Build history of the part. All positions in model axes, mm. A direction names the side the tool comes from. Give positions to 0.01 mm unless a question says otherwise; leave off trailing zeros. Order: outer loops, then holes, each group sorted by start corner. A loop starts at its lowest first (then second) coordinate and runs counter-clockwise, first axis right, second up. Notation, with made-up numbers: (42.5, 3.5) - (82.5, 3.5) arc R26 ccw to (82.5, 38.5) - close; hole circle Ø2 at (33.25, -25.5). An arc over 180 degrees is marked (long way). One line per item, written item: value.
```python
from build123d import *

# Parameters (mm, degrees)
F0_W      = 43.3
F0_H      = 33.3
F1_DEPTH  = 10
F2_W      = 40
F2_H      = 30
F3_DEPTH  = 8.5
F4_W      = 25.5
F4_H      = 15
F5_DEPTH  = 25
F4_R      = 0.85
F6_DEPTH  = 4
F7_W      = 43.3
F7_H      = 33.3
F7_W_2    = 41.7
F7_H_2    = 31.7
F8_DEPTH  = 1
F9_R      = 2
F9_R_2    = 1
F10_DEPTH = 5
F12_SIZE  = 1
F13_R     = 1.3


with BuildPart() as f1:
    # F0 (on Top) → F1 (new body)
    with BuildSketch(Plane.XY):
        Rectangle(F0_W, F0_H)
    extrude(amount=F1_DEPTH)

    # F2 (on face) → F3 (cut)
    with BuildSketch(Plane.XY):
        Rectangle(F2_W, F2_H)
    extrude(amount=F3_DEPTH, mode=Mode.SUBTRACT)

    # F4 (on face) → F5 (cut)
    with BuildSketch(Plane(origin=(0, 0, 8.5), x_dir=(1, 0, 0), z_dir=(0, 0, -1))):
        with Locations((0, -2.1)):
            Rectangle(F4_W, F4_H)
    extrude(amount=-F5_DEPTH, mode=Mode.SUBTRACT)

    # F4 (on face) → F6 (join)
    with BuildSketch(Plane(origin=(0, 0, 8.5), x_dir=(1, 0, 0), z_dir=(0, 0, -1))):
        with Locations((12.2893061021, 12)):
            Circle(F4_R)
        with Locations((-12.2893061021, 12)):
            Circle(F4_R)
        with Locations((-12.2893061021, -12)):
            Circle(F4_R)
        with Locations((12.2893061021, -12)):
            Circle(F4_R)
    extrude(amount=F6_DEPTH)

    # F7 (on face) → F8 (join)
    with BuildSketch(Plane(origin=(0, 0, 0), x_dir=(1, 0, 0), z_dir=(0, 0, -1))):
        Rectangle(F7_W, F7_H)
        Rectangle(F7_W_2, F7_H_2, mode=Mode.SUBTRACT)
    extrude(amount=F8_DEPTH)

    # F9 (on face) → F10 (join)
    with BuildSketch(Plane(origin=(0, 0, 8.5), x_dir=(1, 0, 0), z_dir=(0, 0, -1))):
        with Locations((-17.3809109858, 0)):
            Circle(F9_R)
        with Locations((-17.3809109858, 0)):
            Circle(F9_R_2, mode=Mode.SUBTRACT)
    extrude(amount=F10_DEPTH)

    # F11: F1 across plane


with BuildPart() as f1_1:
    add(f1.part)
    add(f1.part.mirror(Plane.YZ))

    # F12
    f12_edges = [f1_1.edges().sort_by_distance(p)[0] for p in [
        (0, 9.6, 10),
        (-12.75, 2.1, 10),
        (0, -5.4, 10),
        (12.75, 2.1, 10),
    ]]
    chamfer(f12_edges, length=F12_SIZE)

    # F13
    f13_edges = [f1_1.edges().sort_by_distance(p)[0] for p in [
        (-21.65, 16.65, 4.5),
        (21.65, 16.65, 4.5),
        (21.65, -16.65, 4.5),
        (-21.65, -16.65, 4.5),
        (0, -16.65, 10),
        (-21.65, 0, 10),
        (21.65, 0, 10),
        (0, 16.65, 10),
    ]]
    fillet(f13_edges, radius=F13_R)


solid = f1_1.part
```
(1) Slice it at D-D, the plane y = -8.5. Give the cut face in (x, z).
Completed:
outline: (-21.65, -1) - (-20.85, -1) - (-20.85, 0) - (-20, 0) - (-20, 8.5) - (20, 8.5) - (20, 0) - (20.85, 0) - (20.85, -1) - (21.65, -1) - (21.65, 8.7) arc R1.3 ccw to (20.35, 10) - (-20.35, 10) arc R1.3 ccw to (-21.65, 8.7) - close
(2) Pin check, flat tips, straight feed: P1, Ø0.6, axis at x = 17.5, y = 0, coming from the -Z side; P2, Ø0.8, axis at x = 12.5, y = 12, coming from the -Z side; P3, Ø2, axis at x = -17.5, y = 0.5, coming from the -Z side. Stop position of each tip, or through.
Completed:
P1: z = 8.5
P2: z = 4.5
P3: z = 3.5
(3) Drill centre lines: line 1 (X direction, y = 0, z = 7.05); line 2 (Y direction, x = 0, z = 4.25); line 3 (X direction, y = 10, z = 4). Where is each one in solid material? Low to high.
Completed:
line 1: -21.65 to -20, -19.38 to -18.38, -16.38 to -15.38, 15.38 to 16.38, 18.38 to 19.38, 20 to 21.65
line 2: -16.65 to -15, 15 to 16.65
line 3: -21.65 to -20, 20 to 21.65
(4) Slice it at C-C, the plane y = 12. Give the cut face in (x, z).
Completed:
outline: (-21.65, -1) - (-20.85, -1) - (-20.85, 0) - (-20, 0) - (-20, 8.5) - (-13.14, 8.5) - (-13.14, 4.5) - (-11.44, 4.5) - (-11.44, 8.5) - (11.44, 8.5) - (11.44, 4.5) - (13.14, 4.5) - (13.14, 8.5) - (20, 8.5) - (20, 0) - (20.85, 0) - (20.85, -1) - (21.65, -1) - (21.65, 8.7) arc R1.3 ccw to (20.35, 10) - (-20.35, 10) arc R1.3 ccw to (-21.65, 8.7) - close
(5) Slice it at A-A, the plane x = 9.5. Give the cut face in (y, z), and give its area (3 significant figures).
Completed:
outline: (-16.65, -1) - (-15.85, -1) - (-15.85, 0) - (-15, 0) - (-15, 8.5) - (-5.4, 8.5) - (-5.4, 9) - (-6.4, 10) - (-15.35, 10) arc R1.3 ccw to (-16.65, 8.7) - close; (9.6, 8.5) - (15, 8.5) - (15, 0) - (15.85, 0) - (15.85, -1) - (16.65, -1) - (16.65, 8.7) arc R1.3 ccw to (15.35, 10) - (10.6, 10) - (9.6, 9) - close
area: 55.4 mm²
(6) Slice it at B-B, the plane z = 1. Give the cut face in (x, y), and give its area (3 significant figures).
Completed:
outline: (-21.65, -15.35) arc R1.3 ccw to (-20.35, -16.65) - (20.35, -16.65) arc R1.3 ccw to (21.65, -15.35) - (21.65, 15.35) arc R1.3 ccw to (20.35, 16.65) - (-20.35, 16.65) arc R1.3 ccw to (-21.65, 15.35) - close; hole (-20, -15) - (20, -15) - (20, 15) - (-20, 15) - close
area: 240 mm²
(7) 3-axis set-ups, long thin cutter, end or side, ignore diameter. For faces 1 (the face through (0, -7, 10)), 2 (the face through (-12, -12, 4.5)), 3 (the face through (13.24, 1.98, 9.49)): which of +Z, -Z, +X, -X, +Y, -Y reach the whole face in a straight line?
Completed:
face 1: +Z, +X, -X, +Y, -Y
face 2: -Z
face 3: +Z
(8) Pull direction X, two halves, no side cores. Call faces 4 (the face through (0, -16.65, 4)), 5 (the face through (21.26, 16.28, 3.78)), 6 (the face through (-11.832, 11.283, 6.528)): +X half, -X half, draft (parallel to the pull), parting line (faces both ways), or undercut.
Completed:
face 4: draft
face 5: +X half
face 6: undercut
